```python
from build123d import *

# Parameters (mm, degrees)
SKETCH1_W           = 15.88
SKETCH1_H           = 27.7
BOSS_EXTRUDE1_DEPTH = 9.85
SKETCH2_W           = 0.61
SKETCH2_H           = 4.75
SKETCH2_W_2         = 0.43
BOSS_EXTRUDE2_DEPTH = 10
SKETCH4_R           = 1.45
SKETCH4_R_2         = 1.6
CUT_EXTRUDE1_DEPTH  = 10
SKETCH5_W           = 1
SKETCH5_H           = 4.15
BOSS_EXTRUDE3_DEPTH = 3
SKETCH7_R           = 3.362536074
SKETCH7_R_2         = 2.362536074
BOSS_EXTRUDE5_DEPTH = 4.15
CUT_EXTRUDE2_DEPTH  = 43.42645861


with BuildPart() as part:
    # Sketch1 → Boss-Extrude1 (new body)
    with BuildSketch(Plane(origin=(0, 0, 0), x_dir=(1, 0, 0), z_dir=(0, 1, 0))):
        with Locations((7.94, 13.85)):
            Rectangle(SKETCH1_W, SKETCH1_H)
    extrude(amount=BOSS_EXTRUDE1_DEPTH)

    # Sketch2 → Boss-Extrude2 (add)
    with BuildSketch(Plane.XY):
        with Locations((10.185, 4.925)):
            Rectangle(SKETCH2_W, SKETCH2_H)
        with Locations((4.515, 4.925)):
            Rectangle(SKETCH2_W_2, SKETCH2_H)
    extrude(amount=BOSS_EXTRUDE2_DEPTH)

    # Sketch4 → Cut-Extrude1 (cut)
    with BuildSketch(Plane(origin=(0, 9.85, 0), x_dir=(1, 0, 0), z_dir=(0, 1, 0))):
        with Locations(Location((2.82, 2.725, 0), (0, 0, 270))):
            Circle(SKETCH4_R)
        with Locations(Location((12.98, 25, 0), (0, 0, 270))):
            Circle(SKETCH4_R_2)
    extrude(amount=-CUT_EXTRUDE1_DEPTH, mode=Mode.SUBTRACT)

    # Sketch5 → Boss-Extrude3 (add)
    with BuildSketch(Plane.ZY):
        with Locations((-12.2, 4.925)):
            Rectangle(SKETCH5_W, SKETCH5_H)
    extrude(amount=BOSS_EXTRUDE3_DEPTH)

    # Sketch7 → Boss-Extrude5 (add)
    # profile 1 of 2: a face of its own
    with BuildSketch(Plane(origin=(0, 7, 0), x_dir=(1, 0, 0), z_dir=(0, 1, 0))):
        with Locations((-4.220862881, 35.35218968)):
            Circle(SKETCH7_R)
        with Locations((-4.220862881, 35.35218968)):
            Circle(SKETCH7_R_2, mode=Mode.SUBTRACT)
    # profile 2 of 2: a face of its own
    with BuildSketch(Plane(origin=(0, 7, 0), x_dir=(1, 0, 0), z_dir=(0, 1, 0))):
        Polygon((-3, 11.7), (-5, 33), (-4, 33), (-2, 11.7), align=None)
    extrude(amount=-BOSS_EXTRUDE5_DEPTH)

    # Sketch8 → Cut-Extrude2 (cut, through all)
    with BuildSketch(Plane(origin=(0, 2.85, 0), x_dir=(-1, 0, 0), z_dir=(0, -1, 0))):
        Polygon((3.906514494, 32.004379359), (-0.89687697, 32.455402032), (-0.268180196, 39.151022673), (4.535211268, 38.7), align=None)
    extrude(amount=-CUT_EXTRUDE2_DEPTH, mode=Mode.SUBTRACT)


solid = part.part
```
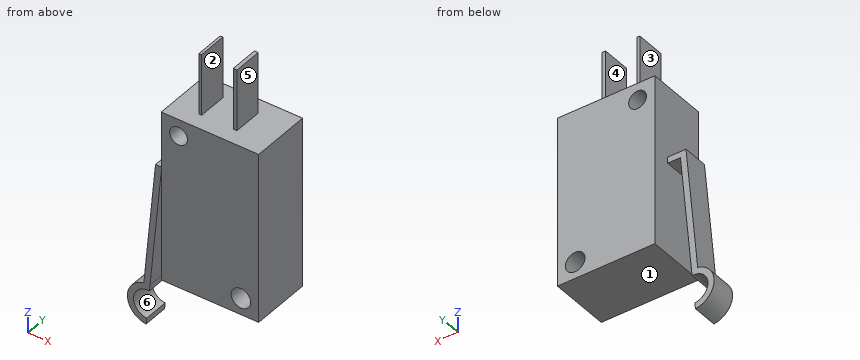
Geometry check sheet. Reference: the model listing, model coordinates, mm. Face numbers are marked on the shaded views. A direction names the side the tool comes from. Round coordinates to 2 decimals unless told otherwise and drop trailing zeros. Loops run counter-clockwise (first coordinate to the right, second up) from the corner with the lowest first, then second, coordinate; pieces in that order, holes last. Notation, with made-up numbers: (2.25, -2) - (60.25, -2) arc R27 cw to (60.25, 22) - close; hole circle Ø1 at (-28.75, 86). An arc over 180 degrees is marked (long way). Use a Markdown table: item, result.
Q1. Material ranges on line 1 (X direction, y = 6.25, z = 7.5); line 2 (Z direction, x = 0.5, y = 4.75); line 3 (X direction, y = 1, z = -2.5), recorded low to high.
Solutions:
| item | result |
|---|---|
| line 1 | x = 4.3 to 4.73, 9.88 to 10.49 |
| line 2 | z = -27.7 to 0 |
| line 3 | x = 0 to 1.39, 4.25 to 15.88 |
Q2. Go/stop test with flat-tipped pins: P1, Ø3, axis at y = 3.5, z = -15.5, coming from the -X side; P2, Ø5, axis at x = 5.5, y = 6, coming from the +Z side; P3, Ø1, axis at x = -1.5, y = 5, coming from the -Z side; P4, Ø4, axis at x = 5.5, y = 3, coming from the -Z side. Record where each tip stops, or that it passes through.
Solutions:
| item | result |
|---|---|
| P1 | stops at x = -3.5 |
| P2 | stops at z = 10 |
| P3 | stops at z = -12.7 |
| P4 | stops at z = -27.7 |
Q3. Cross-section at A-A on x = 2.82. Record the cut outline in (y, z) (3 decimals).
Solutions:
| item | result |
|---|---|
| outline | (0, -27.7) - (9.85, -27.7) - (9.85, -4.175) - (0, -4.175) - close; (0, -1.275) - (9.85, -1.275) - (9.85, 0) - (0, 0) - close |
Q4. Cross-section at D-D on z = -25. Record the cut outline in (x, y), plus the area to 3 significant figures.
Solutions:
| item | result |
|---|---|
| outline | (-4.25, 2.85) - (-3.25, 2.85) - (-3.25, 7) - (-4.25, 7) - close; (0, 0) - (11.38, 0) - (11.38, 9.85) - (0, 9.85) - close; (14.58, 0) - (15.88, 0) - (15.88, 9.85) - (14.58, 9.85) - close |
| area | 129 mm2 |
Q5. Cross-section at B-B on z = 4. Record the cut outline in (x, y), plus the area to 3 significant figures.
Solutions:
| item | result |
|---|---|
| outline | (4.3, 2.55) - (4.73, 2.55) - (4.73, 7.3) - (4.3, 7.3) - close; (9.88, 2.55) - (10.49, 2.55) - (10.49, 7.3) - (9.88, 7.3) - close |
| area | 4.94 mm2 |
Q6. Cross-section at C-C on y = 7.75. Record the cut outline in (x, z) (3 decimals), plus the area to 3 significant figures.
Solutions:
| item | result |
|---|---|
| outline | (0, -27.7) - (15.88, -27.7) - (15.88, 0) - (0, 0) - close; hole circle Ø2.9 at (2.82, -2.725); hole circle Ø3.2 at (12.98, -25) |
| area | 425 mm2 |
Q7. Access from +Z, -Z, +X, -X, +Y, -Y to the whole of each face (thin tool, end or side, straight path). Record for the marked faces 4, 5 and 6.
Solutions:
| item | result |
|---|---|
| face 4 | +Z, +Y, -Y |
| face 5 | +Z, +X, +Y, -Y |
| face 6 | +X, +Y, -Y |
Q8. Draft check along X on the marked faces 1, 2 and 3. Enter one of: released by +X, released by -X, zero draft, split by the parting line, or undercut.
Solutions:
| item | result |
|---|---|
| face 1 | zero draft |
| face 2 | undercut |
| face 3 | released by -X |
